Autodesk Fusion 360 part; units mm, degrees
sketch "スケッチ3" plane through (0, 0, 0) normal (0, 0, 1) x (1, 0, 0)
  line L0 (0, 0) -> (45, 0)
  line L1 (45, 0) -> (45, 9)
  line L2 (45, 9) -> (0, 9)
  line L3 (0, 9) -> (0, 0)
  dimension "d4" = 45
  dimension "d5" = 9
extrude "押し出し2" add sketch "スケッチ3" along normal blind 5.8
sketch "スケッチ4" plane through (0, 0, 0) normal (1, 0, 0) x (0, 1, 0)
sketch "スケッチ5" plane through (45, 0, 0) normal (1, 0, 0) x (0, 1, 0)
  line L0 (0, 0) -> (9, 0)
  line L1 (9, 0) -> (9, 5.8)
  line L2 (9, 5.8) -> (0, 5.8)
  line L3 (0, 5.8) -> (0, 0)
  line L4 (0, 0) -> (0.85, 0)
  line L5 (0.85, 0) -> (0.85, 5.8)
  line L6 (0.85, 5.8) -> (0, 5.8)
  line L7 (0, 5.8) -> (0, 0)
  line L8 (9, 0) -> (8.15, 0)
  line L9 (8.15, 0) -> (8.15, 5.7622)
  line L10 (8.15, 5.7622) -> (9, 5.7622)
  line L11 (9, 5.7622) -> (9, 0)
  line L12 (0.85, 0) -> (8.15, 0)
  line L13 (8.15, 0) -> (8.15, 1)
  line L14 (8.15, 1) -> (0.85, 1)
  line L15 (0.85, 1) -> (0.85, 0)
  line L16 (0.85, 5.8) -> (8.1927, 5.8)
  line L17 (8.1927, 5.8) -> (8.1927, 1.8)
  line L18 (8.1927, 1.8) -> (0.85, 1.8)
  line L19 (0.85, 1.8) -> (0.85, 5.8)
  line L20 (4.5, 1) -> (6.55, 1)
  line L21 (6.55, 1) -> (6.55, 0)
  line L22 (6.55, 0) -> (4.5, 0)
  line L23 (4.5, 0) -> (4.5, 1)
  line L24 (4.5, 0) -> (2.45, 0)
  line L25 (2.45, 0) -> (2.45, 1)
  line L26 (2.45, 1) -> (4.5, 1)
  line L27 (4.5, 1) -> (4.5, 0)
  dimension "d8" = 0.85
  dimension "d9" = 0.85
  dimension "d10" = 1
  dimension "d11" = 4
  dimension "d12" = 2.05
  dimension "d13" = 2.05
sketch "スケッチ6" plane through (0, 0, 5.8) normal (0, 0, 1) x (-1, 0, 0)
  line L0 (0, -9) -> (0, 0)
  line L1 (0, 0) -> (-45, 0)
  line L2 (-45, 0) -> (-45, -9)
  line L3 (-45, -9) -> (0, -9)
  line L4 (-45, -9) -> (-17.5, -9)
  line L5 (-17.5, -9) -> (-17.5, -4.5)
  line L6 (-17.5, -4.5) -> (-45, -4.5)
  line L7 (-45, -4.5) -> (-45, -9)
  circle A0 centre (-17.5, -4.5) radius 3.2
  dimension "d16" = 27.5
  dimension "d17" = 4.5
  dimension "d18" = 6.4
extrude "押し出し4" cut sketch "スケッチ6" against normal blind 9 contours L5 L6 A0 | L5 L6 A0
sketch "スケッチ7" plane through (0, 0, 0) normal (-1, 0, 0) x (0, -1, 0)
  line L0 (-9, 0) -> (0, 0)
  line L1 (0, 0) -> (0, 5.8)
  line L2 (0, 5.8) -> (-9, 5.8)
  line L3 (-9, 5.8) -> (-9, 0)
  line L4 (-9, 0) -> (0, 5.8)
  line L5 (-9, 5.8) -> (0, 0)
  circle A0 centre (-4.5, 2.9) radius 1
  dimension "d21" = 2
extrude "押し出し5" cut sketch "スケッチ7" against normal blind 15 contours L4 L5 A0 | L4 L5 A0 | L4 L5 A0 | L4 L5 A0
sketch "スケッチ8" plane through (0, 0, 0) normal (-1, 0, 0) x (0, -1, 0)
  circle A0 centre (-4.5, 2.9) radius 1
  line L0 (-9, 0) -> (0, 0)
  line L1 (0, 0) -> (0, 5.8)
  line L2 (0, 5.8) -> (-9, 5.8)
  line L3 (-9, 5.8) -> (-9, 0)
  circle A1 centre (-4.5, 2.9) radius 1.55
  dimension "d24" = 3.1
extrude "押し出し6" cut sketch "スケッチ8" against normal blind 4 contours A1
sketch "スケッチ9" plane through (45, 0, 0) normal (1, 0, 0) x (0, 1, 0)
  line L0 (9, 0) -> (9, 5.8)
  line L1 (9, 5.8) -> (0, 5.8)
  line L2 (0, 5.8) -> (0, 0)
  line L3 (0, 0) -> (9, 0)
sketch "スケッチ10" plane through (45, 0, 0) normal (1, 0, 0) x (0, 1, 0)
  line L0 (0, 0) -> (9, 0)
  line L1 (9, 0) -> (9, 5.8)
  line L2 (9, 5.8) -> (0, 5.8)
  line L3 (0, 5.8) -> (0, 0)
extrude "押し出し7" add sketch "スケッチ9" along normal blind 10
sketch "スケッチ11" plane through (55, 0, 0) normal (1, 0, 0) x (0, 1, 0)
  line L0 (0, 0) -> (9, 0)
  line L1 (9, 0) -> (9, 5.8)
  line L2 (9, 5.8) -> (0, 5.8)
  line L3 (0, 5.8) -> (0, 0)
  line L4 (0, 0) -> (4.5, 0)
  line L5 (4.5, 0) -> (6.55, 0)
  line L6 (6.55, 0) -> (6.55, 1)
  line L7 (6.55, 1) -> (4.5, 1)
  line L8 (4.5, 1) -> (4.5, 0)
  line L9 (4.5, 0) -> (2.45, 0)
  line L10 (2.45, 0) -> (2.45, 1)
  line L11 (2.45, 1) -> (4.5, 1)
  line L12 (4.5, 1) -> (4.5, 0)
  line L13 (9, 0) -> (8.3, 0)
  line L14 (8.3, 0) -> (8.3, 5.8)
  line L15 (8.3, 5.8) -> (9, 5.8)
  line L16 (9, 5.8) -> (9, 0)
  line L17 (0, 0) -> (0.7, 0)
  line L18 (0.7, 0) -> (0.7, 5.8)
  line L19 (0.7, 5.8) -> (0, 5.8)
  line L20 (0, 5.8) -> (0, 0)
  line L21 (0.7, 1) -> (8.3, 1)
  line L22 (8.3, 1) -> (8.3, 1.9)
  line L23 (8.3, 1.9) -> (0.7, 1.9)
  line L24 (0.7, 1.9) -> (0.7, 1)
  line L25 (4.5, 1.9) -> (6.55, 1.9)
  line L26 (6.55, 1.9) -> (6.55, 4.9)
  line L27 (6.55, 4.9) -> (4.5, 4.9)
  line L28 (4.5, 4.9) -> (4.5, 1.9)
  line L29 (4.5, 1.9) -> (2.45, 1.9)
  line L30 (2.45, 1.9) -> (2.45, 4.9)
  line L31 (2.45, 4.9) -> (4.5, 4.9)
  line L32 (4.5, 4.9) -> (4.5, 1.9)
  dimension "d29" = 4.5
  dimension "d30" = 2.05
  dimension "d31" = 1
  dimension "d32" = 0.9
  dimension "d33" = 2.05
  dimension "d34" = 3
  dimension "d35" = 2.05
extrude "押し出し8" cut sketch "スケッチ11" against normal blind 28 contours L0 L4 L8 L9 L10 L11 L12 L21 | L7 L11 L14 L18 L21 L22 L23 L24 L25 L29 | L0 L5 L6 L7 L8 L12 L21 | L23 L28 L29 L30 L31 L32 | L23 L25 L26 L27 L28 L32
sketch "スケッチ12" plane through (0, 0, 4.9) normal (0, 0, -1) x (1, 0, 0)
  line L0 (55, -6.55) -> (55, -2.45)
  line L1 (55, -2.45) -> (27, -2.45)
  line L2 (27, -2.45) -> (27, -6.55)
  line L3 (27, -6.55) -> (55, -6.55)
  line L4 (55, -6.55) -> (27, -6.55)
  line L5 (27, -6.55) -> (27, -2.45)
  line L6 (27, -2.45) -> (55, -2.45)
  line L7 (55, -2.45) -> (55, -6.55)
extrude "押し出し9" add sketch "スケッチ12" along normal blind 1.2
Verification items for the finished model (mm, model axes). A direction names the side the tool comes from. Give positions to 0.01 mm unless a question says otherwise; leave off trailing zeros. Order: outer loops, then holes, each group sorted by start corner. A loop starts at its lowest first (then second) coordinate and runs counter-clockwise, first axis right, second up. Notation, with made-up numbers: (-12, -6) -> (13, -6) arc R22 cw to (13, 2) -> close; hole circle Ø7 at (-34.75, -3.75). An arc over 180 degrees is marked (long way). Answer as CSV lines item,"result".
Q1. Access from +Z, -Z, +X, -X, +Y, -Y to the whole of each face (thin tool, end or side, straight path). Record for faces 4 (the flat face through (4, 5, 4)), 5 (the flat face through (41, 2, 1.9)), 6 (the flat face through (41.2, 2.45, 0.5)), 7 (the flat face through (0, 6, 2)), 8 (the flat face through (27, 0, 3)).
Solutions:
face 4,"-X"
face 5,"+X"
face 6,"-Z, +X"
face 7,"+Z, -Z, -X, +Y, -Y"
face 8,"+Z, -Z, +X, -X, -Y"
Q2. Sectioned sample at A-A on z = 0.55. Record the cut outline in (x, y), plus the area to 3 significant figures.
Solutions:
outline,"(0, 0) -> (55, 0) -> (55, 2.45) -> (27, 2.45) -> (27, 6.55) -> (55, 6.55) -> (55, 9) -> (0, 9) -> close; hole circle Ø6.4 at (17.5, 4.5)"
area,"348 mm²"
Q3. Sectioned sample at B-B on x = 17.5. Record the cut outline in (y, z).
Solutions:
outline,"(0, 0) -> (1.3, 0) -> (1.3, 5.8) -> (0, 5.8) -> close; (7.7, 0) -> (9, 0) -> (9, 5.8) -> (7.7, 5.8) -> close"
Q4. Depth check by flat-ended pin: pin 1 (1.1 mm diameter, centred on x = 41.5, z = 0.5, fed in from -Y). Enter the tip coordinate at first touch or a pass-through.
Solutions:
pin 1,"stops at y = 0"
Q5. Sectioned sample at C-C on y = 4.5. Record the cut outline in (x, z).
Solutions:
outline,"(0, 0) -> (14.3, 0) -> (14.3, 1.9) -> (4, 1.9) -> (4, 1.35) -> (0, 1.35) -> close; (0, 4.45) -> (4, 4.45) -> (4, 3.9) -> (14.3, 3.9) -> (14.3, 5.8) -> (0, 5.8) -> close; (20.7, 0) -> (27, 0) -> (27, 3.7) -> (55, 3.7) -> (55, 5.8) -> (20.7, 5.8) -> close"
Q6. Sectioned sample at D-D on y = 7. Record the cut outline in (x, z).
Solutions:
outline,"(0, 0) -> (15.5, 0) -> (15.5, 5.8) -> (0, 5.8) -> close; (19.5, 0) -> (55, 0) -> (55, 1) -> (27, 1) -> (27, 1.9) -> (55, 1.9) -> (55, 5.8) -> (19.5, 5.8) -> close"
Q7. Release check for a two-part mould opening along X. For faces 1 (the cylindrical face through (20.7, 4.4, 2.9)), 2 (the flat face through (55, 5, 4)), 3 (the flat face through (41, 2, 1)) record: +X half, -X half, draft (parallel to the pull), parting line (faces both ways), or undercut.
Solutions:
face 1,"undercut"
face 2,"+X half"
face 3,"draft"
Q8. Scan lines: probe 1 along Z at (x, y) = (47, 7.75); probe 2 along Z at (x, y) = (6.5, 4.5); probe 3 along Y at (x, z) = (10.5, 2.9). Record each from-to range of solid material in increasing order.
Solutions:
probe 1,"z = 0 to 1, 1.9 to 5.8"
probe 2,"z = 0 to 1.9, 3.9 to 5.8"
probe 3,"y = 0 to 3.5, 5.5 to 9"
